Check sheet for the modelled part. Datum: model origin and axes. Units: mm. Face numbers are marked on the shaded views. A direction names the side the tool comes from. Give positions to 0.01 mm unless a question says otherwise; leave off trailing zeros. Write each loop counter-clockwise with the first axis right and the second up, starting at its lowest first coordinate (ties: lowest second). Pieces come first, ordered by that corner, then holes. Notation, with made-up numbers: M 73.25,44.25 L 125.25,44.25 A23 ccw 125.25,78.25 Z; hole C 4,87.25 d11. An arc over 180 degrees is marked long. One line per item, written item: value. Start each with the question number.
from build123d import *

# Parameters (mm, degrees)
BOSS_EXTRUDE1_START    = -1
SKETCH2_R              = 3.9
BOSS_EXTRUDE1_DEPTH    = 5
M3_CLEARANCE_HOLE1_D   = 3.2
M3_TAPPED_HOLE1_REACH  = 24.345
M3_TAPPED_HOLE1_BORE_R = 1.25
MIRROR3_START          = -6
MIRROR3_OUTLINE_R      = 3.9
MIRROR3_OUTLINE_R_2    = 1.6
MIRROR3_DEPTH          = 5
MIRROR3_START_2        = -6.9
MIRROR3_2_OUTLINE_R    = 1.25
MIRROR3_2_DEPTH        = 3.205747808


with BuildPart() as part:
    # Sketch2 → Boss-Extrude1 (new body)
    with BuildSketch(Plane(origin=(0, 0, 0), x_dir=(0, 0, -1), z_dir=(1, 0, 0)).offset(BOSS_EXTRUDE1_START)):
        with BuildLine():
            Line((2.5, -6.9), (-2.5, -6.9))
            ThreePointArc((-2.5, -6.9), (-3.563882529, -6.593562507), (-4.301751563, -5.768153965))
            ThreePointArc((-4.301751563, -5.768153965), (-4.613436828, -5.232032538), (-5.004243793, -4.750530924))
            ThreePointArc((-5.004243793, -4.750530924), (-6.093212803, -3.237708717), (-6.737511079, -1.488604871))
            Line((-6.737511079, -1.488604871), (-9.185849324, 9.592714537))
            ThreePointArc((-9.185849324, 9.592714537), (-7.820620852, 12.799917558), (-4.343824749, 12.551142838))
            Line((-4.343824749, 12.551142838), (4.399145444, 5.315780221))
            ThreePointArc((4.399145444, 5.315780221), (6.88756759, 0.414020163), (5.004243793, -4.750530924))
            ThreePointArc((5.004243793, -4.750530924), (4.613436828, -5.232032538), (4.301751563, -5.768153965))
            ThreePointArc((4.301751563, -5.768153965), (3.563882529, -6.593562507), (2.5, -6.9))
        make_face()
        Circle(SKETCH2_R, mode=Mode.SUBTRACT)
    extrude(amount=BOSS_EXTRUDE1_DEPTH)

    # M3 Clearance Hole1 (through all)
    with Locations(Plane.ZY.offset(1)):
        with Locations((6.256496681, 10.239934047)):
            Hole(M3_CLEARANCE_HOLE1_D / 2)

    # M3 Tapped Hole1 bore → M3 Tapped Hole1 (cut, up to next)
    with BuildSketch(Plane(origin=(0, -6.9, 1.914772396), x_dir=(-1, 0, 0), z_dir=(0, -1, 0)), mode=Mode.PRIVATE) as m3_tapped_hole1_sk1:
        with Locations((-2, 1.914772396)):
            Circle(M3_TAPPED_HOLE1_BORE_R)
    m3_tapped_hole1_tool1 = extrude(m3_tapped_hole1_sk1.sketch, amount=-M3_TAPPED_HOLE1_REACH, mode=Mode.PRIVATE) & part.part
    add(m3_tapped_hole1_tool1.solids().sort_by_distance((2, -6.9, 0))[0], mode=Mode.SUBTRACT)

    # Mirror3: read off the stored shape, not the designer's step
    # Mirror3 outline → Mirror3 (add)
    with BuildSketch(Plane.YZ.offset(MIRROR3_START)):
        with BuildLine():
            ThreePointArc((-4.750530924, -5.004243793), (0.414020162, -6.88756759), (5.315780221, -4.399145444))
            Line((5.315780221, -4.399145444), (12.551142838, 4.343824749))
            ThreePointArc((12.551142838, 4.343824749), (12.799917558, 7.820620852), (9.592714537, 9.185849324))
            Line((9.592714537, 9.185849324), (-1.488604871, 6.737511079))
            ThreePointArc((-1.488604871, 6.737511079), (-3.237708717, 6.093212803), (-4.750530924, 5.004243793))
            ThreePointArc((-4.750530924, 5.004243793), (-5.232032538, 4.613436828), (-5.768153965, 4.301751563))
            ThreePointArc((-5.768153965, 4.301751563), (-6.593562507, 3.563882529), (-6.9, 2.5))
            Line((-6.9, 2.5), (-6.9, -2.5))
            ThreePointArc((-6.9, -2.5), (-6.593562507, -3.563882529), (-5.768153965, -4.301751563))
            ThreePointArc((-5.768153965, -4.301751563), (-5.232032538, -4.613436828), (-4.750530924, -5.004243793))
        make_face()
        Circle(MIRROR3_OUTLINE_R, mode=Mode.SUBTRACT)
        with Locations((10.239934047, 6.256496681)):
            Circle(MIRROR3_OUTLINE_R_2, mode=Mode.SUBTRACT)
    extrude(amount=MIRROR3_DEPTH)

    # Mirror3 2 outline → Mirror3 2 (cut)
    with BuildSketch(Plane(origin=(0, 0, 0), x_dir=(1, 0, 0), z_dir=(0, 1, 0)).offset(MIRROR3_START_2)):
        with Locations((-4, 0)):
            Circle(MIRROR3_2_OUTLINE_R)
    extrude(amount=MIRROR3_2_DEPTH, mode=Mode.SUBTRACT)


solid = part.part
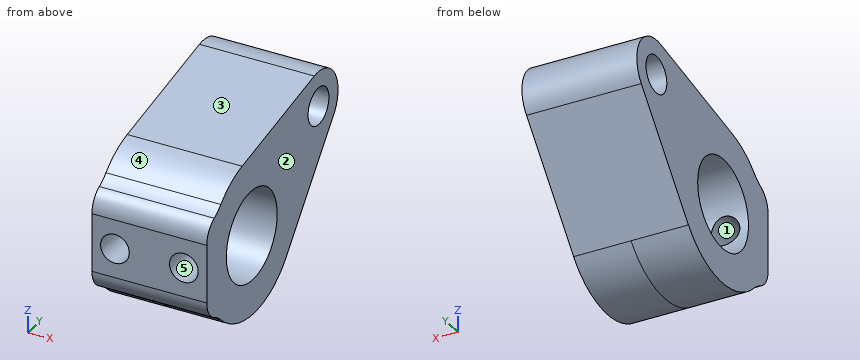
1) Tool access check on the marked faces 4 and 5. Record the directions out of +Z, -Z, +X, -X, +Y, -Y that give a thin tool (end or side, any length) a straight path to the whole face; none if there is none.
2) Gauge pin test, flat ends, axial feed: pin 1 (3 mm diameter, centred on x = 2, z = 0, fed in from +Y); pin 2 (1.9 mm diameter, centred on y = 10.24, z = 6.26, fed in from -X); pin 3 (6 mm diameter, centred on x = 3, y = 8.5, fed in from -Z); pin 4 (4 mm diameter, centred on x = -2.5, y = 6.5, fed in from -Z). Record the tip position at first contact, or that the pin passes through.
3) Draft check along Z on the marked faces 1, 2 and 3. Enter one of: released by +Z, released by -Z, zero draft, split by the parting line, or undercut.
4) Cross-section at D-D (x = -4). Record the boundary of the cut face in (y, z), plus the area to 3 significant figures.
5) Cross-section at A-A (y = 9.25). Record the boundary of the cut face in (x, z), plus the area to 3 significant figures.
6) Material ranges on L1, parallel to X at y = -5.8, z = 0; L2, parallel to Y at x = -5.25, z = 5.5; L3, parallel to Z at x = -0.5, y = 3, recorded low to high. Write a range as from..to.
7) Cross-section at C-C (x = 0.5). Record the boundary of the cut face in (y, z), plus the area to 3 significant figures.
Data:
1. face 4: +Z, +X, -X, -Y
1. face 5: -Y
2. pin 1: stops at y = 10.2
2. pin 2: passes through
2. pin 3: stops at z = -4.18
2. pin 4: stops at z = -5.23
3. face 1: undercut
3. face 2: zero draft
3. face 3: released by +Z
4. outline: M -6.9,-2.5 A2 ccw -5.77,-4.3 A4 cw -4.75,-5 A6.9 ccw 5.32,-4.4 L 12.55,4.34 A3 ccw 9.59,9.19 L -1.49,6.74 A6.9 ccw -4.75,5 A4 cw -5.77,4.3 A2 ccw -6.9,2.5 L -6.9,1.25 L -3.69,1.25 A3.9 cw long -3.69,-1.25 L -6.9,-1.25 Z; hole C 10.24,6.26 d3.2
4. area: 154 mm2
5. outline: M -6,0.35 L 4,0.35 L 4,5 L -6,5 Z; M -6,7.51 L 4,7.51 L 4,9.11 L -6,9.11 Z
5. area: 62.4 mm2
6. L1: x = -6..-5.25, -2.75..0.75, 3.25..4
6. L2: y = -4.17..8.83, 11.65..13.14
6. L3: z = -6.21..-2.49, 2.49..7.73
7. outline: M -6.9,-2.5 A2 ccw -5.77,-4.3 A4 cw -4.75,-5 A6.9 ccw 5.32,-4.4 L 12.55,4.34 A3 ccw 9.59,9.19 L -1.49,6.74 A6.9 ccw -4.75,5 A4 cw -5.77,4.3 A2 ccw -6.9,2.5 Z; hole C 0,0 d7.8; hole C 10.24,6.26 d3.2
7. area: 161 mm2
